Verification items for this drawing (mm, ordinates from the low corner). A direction names the side the tool comes from. Round coordinates to 2 decimals unless told otherwise and drop trailing zeros. Write each loop counter-clockwise with the first axis right and the second up, starting at its lowest first coordinate (ties: lowest second). Pieces come first, ordered by that corner, then holes. Notation, with made-up numbers: (88.5, 42) -> (104.5, 42) arc R15 cw to (104.5, 61) -> close; hole circle Ø8 at (65, -0.5). An arc over 180 degrees is marked (long way). Use one line per item in the form item = value. Start each with the question number.
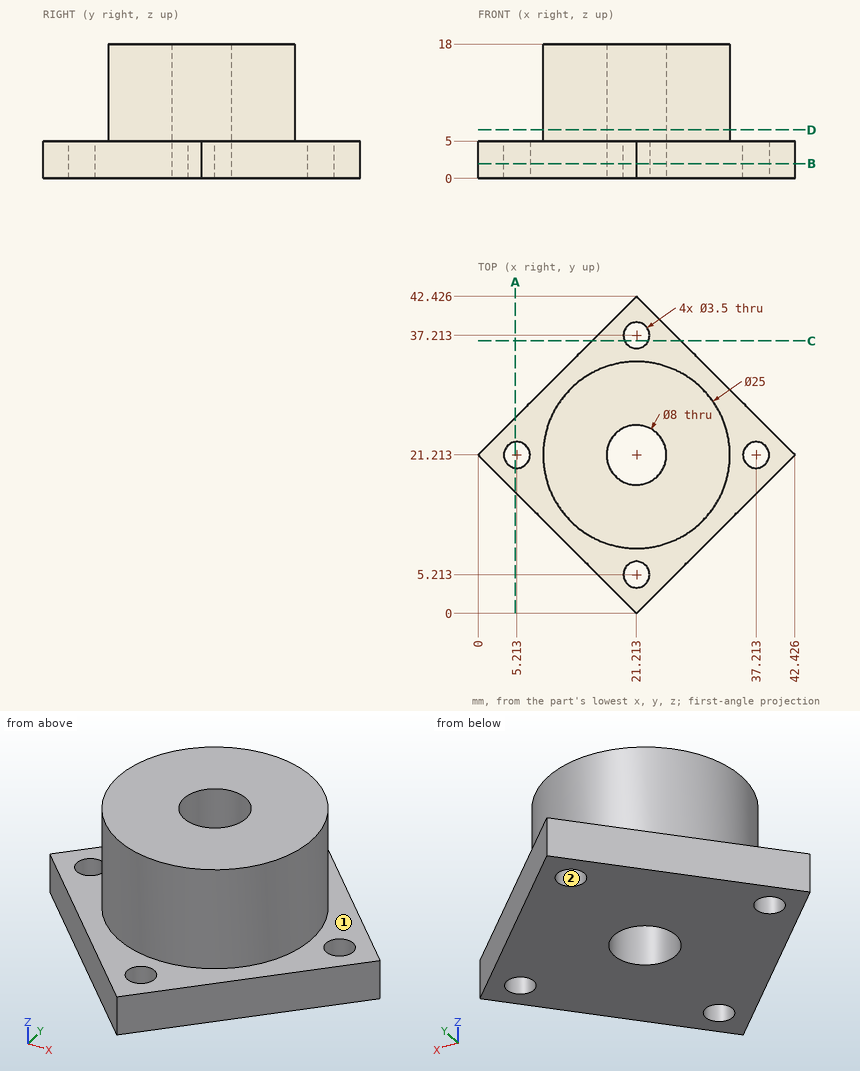
1. Sectioned sample at B-B (z = 2). Enter the section's corners in (x, y).
2. Sectioned sample at A-A (x = 5). Enter the section's corners in (y, z).
3. Scan lines: probe 1 along X at (y, z) = (21.5, 11); probe 2 along Z at (x, y) = (17.5, 6); probe 3 along X at (y, z) = (22, 9.5) (1 decimal). Record each from-to range of solid material in increasing order.
4. Depth check by flat-ended pin: pin 1 (4 mm diameter, centred on x = 21.21, y = 37.21, fed in from +Z); pin 2 (10 mm diameter, centred on x = 20, z = 10.5, fed in from -Y); pin 3 (2 mm diameter, centred on x = 18, z = 8.5, fed in from +Y). Enter the tip coordinate at first touch or a pass-through.
5. Tool access check on the marked faces 1 and 2. Record the directions out of +Z, -Z, +X, -X, +Y, -Y that give a thin tool (end or side, any length) a straight path to the whole face; none if there is none.
6. Sectioned sample at D-D (z = 6.5). Enter the section's corners in (x, y).
7. Sectioned sample at C-C (y = 36.5). Enter the section's corners in (x, z) (1 decimal), and give its area (3 significant figures).
Returned:
q1.outline = (0, 21.21) -> (21.21, 0) -> (42.43, 21.21) -> (21.21, 42.43) -> close; hole circle Ø3.5 at (5.21, 21.21); hole circle Ø8 at (21.21, 21.21); hole circle Ø3.5 at (21.21, 5.21); hole circle Ø3.5 at (21.21, 37.21); hole circle Ø3.5 at (37.21, 21.21)
q2.outline = (16.21, 0) -> (19.48, 0) -> (19.48, 5) -> (16.21, 5) -> close; (22.95, 0) -> (26.21, 0) -> (26.21, 5) -> (22.95, 5) -> close
q3.probe_1 = 8.72 to 17.22, 25.2 to 33.71
q3.probe_2 = 0 to 5
q3.probe_3 = 8.7 to 17.3, 25.1 to 33.7
q4.pin_1 = 5
q4.pin_2 = 8.71
q4.pin_3 = 33.52
q5.face_1 = +Z
q5.face_2 = +Z, -Z
q6.outline = circle Ø25 at (21.21, 21.21); hole circle Ø8 at (21.21, 21.21)
q7.outline = (15.3, 0) -> (19.6, 0) -> (19.6, 5) -> (15.3, 5) -> close; (22.8, 0) -> (27.1, 0) -> (27.1, 5) -> (22.8, 5) -> close
q7.area = 43.3 mm^2
